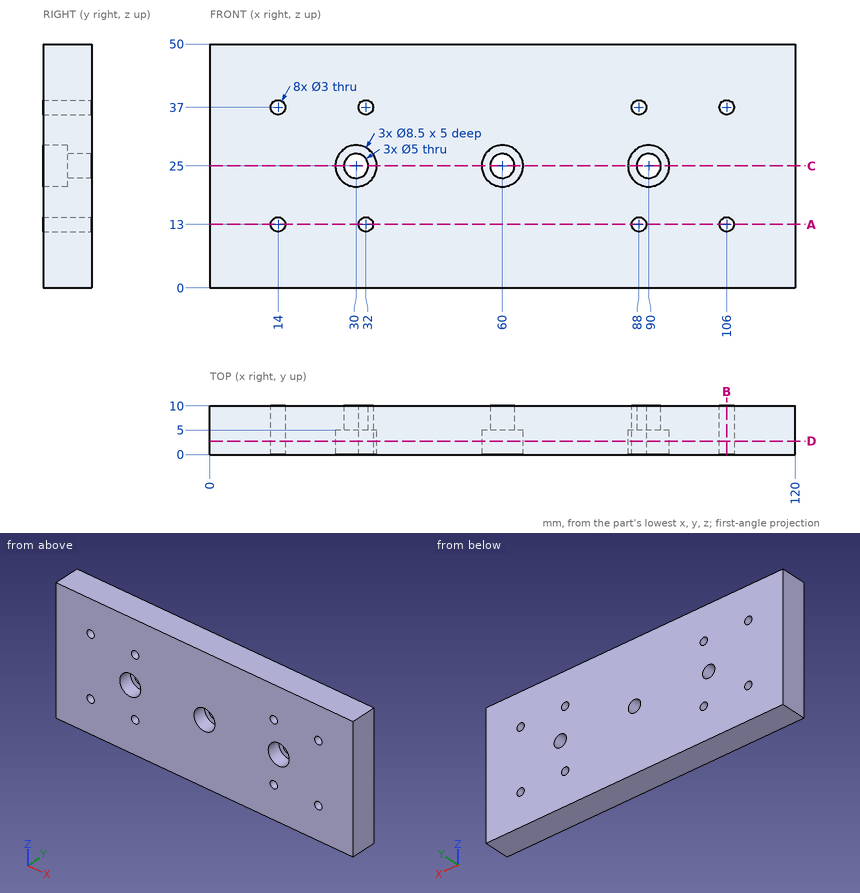
Answer from the drawing. Dimensions are ordinates in mm from the lowest x, y and z of the part. Give positions to 0.01 mm unless a question says otherwise; leave off trailing zeros. Write each loop counter-clockwise with the first axis right and the second up, starting at its lowest first coordinate (ties: lowest second). Pieces come first, ordered by that corner, then holes.
1) Section B-B (x = 106) is taken. Write down the section's boundary in (y, z), and give its area (3 significant figures).
2) Section A-A (z = 13) is taken. Write down the section's boundary in (x, y).
3) Section C-C (z = 25) is taken. Write down the section's boundary in (x, y).
4) Given P1, Ø4, axis at x = 106, z = 13, coming from the +Y side; P2, Ø7, axis at x = 60, z = 25, coming from the -Y side, each flat-ended and moving along its own axis, determine where each tip first touches the part or whether it passes through.
5) Find the intervals of material crossed by L1, parallel to X at y = 3, z = 37; L2, parallel to Z at x = 106, y = 7; L3, parallel to Z at x = 90, y = 1.3, in increasing order.
6) Section D-D (y = 2.75) is taken. Count the separate pieces of the cut face and the enclosed holes in it, and give its area (3 significant figures).
Response:
1. outline: (0, 0) - (10, 0) - (10, 11.5) - (0, 11.5) - close; (0, 14.5) - (10, 14.5) - (10, 35.5) - (0, 35.5) - close; (0, 38.5) - (10, 38.5) - (10, 50) - (0, 50) - close
1. area: 440 mm2
2. outline: (0, 0) - (12.5, 0) - (12.5, 10) - (0, 10) - close; (15.5, 0) - (30.5, 0) - (30.5, 10) - (15.5, 10) - close; (33.5, 0) - (86.5, 0) - (86.5, 10) - (33.5, 10) - close; (89.5, 0) - (104.5, 0) - (104.5, 10) - (89.5, 10) - close; (107.5, 0) - (120, 0) - (120, 10) - (107.5, 10) - close
3. outline: (0, 0) - (25.75, 0) - (25.75, 5) - (27.5, 5) - (27.5, 10) - (0, 10) - close; (32.5, 5) - (34.25, 5) - (34.25, 0) - (55.75, 0) - (55.75, 5) - (57.5, 5) - (57.5, 10) - (32.5, 10) - close; (62.5, 5) - (64.25, 5) - (64.25, 0) - (85.75, 0) - (85.75, 5) - (87.5, 5) - (87.5, 10) - (62.5, 10) - close; (92.5, 5) - (94.25, 5) - (94.25, 0) - (120, 0) - (120, 10) - (92.5, 10) - close
4. P1: stops at y = 10
4. P2: stops at y = 5
5. L1: x = 0 to 12.5, 15.5 to 30.5, 33.5 to 86.5, 89.5 to 104.5, 107.5 to 120
5. L2: z = 0 to 11.5, 14.5 to 35.5, 38.5 to 50
5. L3: z = 0 to 20.75, 29.25 to 50
6. separate pieces: 1
6. enclosed holes: 11
6. area: 5,770 mm2
